```python
from build123d import *

# Parameters (mm, degrees)
SKETCH1_W           = 249.6
SKETCH1_H           = 267.4
BOSS_EXTRUDE1_DEPTH = 5
SKETCH5_W           = 249.6
SKETCH5_H           = 131.304588604
CUT_EXTRUDE3_DEPTH  = 6


with BuildPart() as part:
    # Sketch1 → Boss-Extrude1 (new body)
    with BuildSketch(Plane.XY):
        with Locations((124.8, -133.7)):
            Rectangle(SKETCH1_W, SKETCH1_H)
    extrude(amount=BOSS_EXTRUDE1_DEPTH)

    # Sketch5 → Cut-Extrude3 (cut, through all)
    with BuildSketch(Plane.XY.offset(5)):
        with Locations((124.8, -201.747705698)):
            Rectangle(SKETCH5_W, SKETCH5_H)
        with BuildLine():
            Line((249.6, 25), (206.197139999, 25))
            ThreePointArc((206.197139999, 25), (143.697139999, -37.5), (206.197139999, -100))
            Line((206.197139999, -100), (249.6, -100))
            Line((249.6, -100), (249.6, 25))
        make_face()
        with BuildLine():
            Line((0, 25), (0, -100))
            Line((0, -100), (43.402860001, -100))
            ThreePointArc((43.402860001, -100), (105.902860001, -37.5), (43.402860001, 25))
            Line((43.402860001, 25), (0, 25))
        make_face()
    extrude(amount=-CUT_EXTRUDE3_DEPTH, mode=Mode.SUBTRACT)


solid = part.part
```
Geometry check sheet. Reference: the model listing, model coordinates, mm. A direction names the side the tool comes from. Round coordinates to 2 decimals unless told otherwise and drop trailing zeros. Loops run counter-clockwise (first coordinate to the right, second up) from the corner with the lowest first, then second, coordinate; pieces in that order, holes last. Notation, with made-up numbers: M 59.25,28.5 L 91.25,28.5 A23 cw 91.25,37.5 Z; hole C 36,36.25 d3. An arc over 180 degrees is marked long. Return JSON: item names as keys, results as strings. Group by question number.
(1) Set-up check for faces 4 (the face through (249.6, -118, 2)), 5 (the face through (228, -100, 3)): record each of +Z, -Z, +X, -X, +Y, -Y from which the full face is reachable in a straight line by a thin tool's end or side.
(2) Section check C-C, the plane y = -51.5. Enter the section's corners in (x, z), and give its area (3 significant figures).
(3) Section check B-B, the plane x = 226. Enter the section's corners in (y, z), and give its area (3 significant figures).
(4) Mould release check, pull along Y, two halves, no side actions. Record for faces 1 (the face through (123, -97, 5)), 2 (the face through (98.865, -66.314, 2.535)), 3 (the face through (21, -100, 3)): pulls with the +Y half, pulls with the -Y half, needs draft (parallel to the pull), parting line crosses it, or undercut.
(5) Section check A-A, the plane z = 1.6. Enter the section's corners in (x, y).
(6) Scan lines: line 1 along Y through (x, z) = (151, 4.2); line 2 along Y through (x, z) = (33, 1.95); line 3 along X through (y, z) = (-11.5, 1.85). Record each from-to range of solid material in increasing order. Write a range as [from, to].
(7) Go/stop test with flat-tipped pins: pin 1 (2 mm diameter, centred on x = 85.5, z = 3.5, fed in from +Y); pin 2 (1.5 mm diameter, centred on x = 228.5, z = 3.5, fed in from +Y); pin 3 (2 mm diameter, centred on x = 30, y = -106, fed in from -Z); pin 4 (1.5 mm diameter, centred on y = -71, z = 1, fed in from +X). Record where each tip stops, or that it passes through.
Data:
{
 "1": {"face 4": "+Z, -Z, +X, +Y, -Y", "face 5": "+Z, -Z, +X, +Y"},
 "2": {"outline": "M 104.31,0 L 145.29,0 L 145.29,5 L 104.31,5 Z", "area": "205 mm²"},
 "3": {"outline": "M -136.1,0 L -100,0 L -100,5 L -136.1,5 Z", "area": "180 mm²"},
 "4": {"face 1": "needs draft", "face 2": "undercut", "face 3": "pulls with the +Y half"},
 "5": {"outline": "M 0,-136.1 L 249.6,-136.1 L 249.6,-100 L 206.2,-100 A62.5 cw 156.2,0 L 93.4,0 A62.5 cw 43.4,-100 L 0,-100 Z"},
 "6": {"line 1": "[-136.1, -66.82], [-8.18, 0]", "line 2": "[-136.1, -100]", "line 3": "[100.24, 149.36]"},
 "7": {"pin 1": "y = -82.76", "pin 2": "y = -100", "pin 3": "z = 0", "pin 4": "x = 153.92"}
}
